Answer from the drawing. Dimensions are ordinates in mm from the lowest x, y and z of the part. Coordinates: 2 decimals unless noted, no trailing zeros. Write each loop counter-clockwise with the first axis right and the second up, starting at its lowest first coordinate (ties: lowest second). Pieces come first, ordered by that corner, then holes.
1) Each of these flat-tipped pins is pushed along its axis until it touches: pin 1 Ø1.5 at (y, z) = (1, 51.5) entering from +X; pin 2 Ø0.9 at (y, z) = (1.5, 51.5) entering from -X. Where does it stop, or does it pass through?
2) Find the intervals of material crossed by line 1 (X direction, y = 0.35, z = 23); line 2 (Z direction, x = 22.5, y = 0.25); line 3 (Z direction, x = 6.5, y = 1.55), in increasing order.
3) The part is cut by section A-A (x = 5.5). Determine the outline of the cut face in (y, z), then the cut area to 3 significant figures.
4) The part is cut by section B-B (z = 38). Determine the outline of the cut face in (x, y).
5) The part is cut by section C-C (y = 2.4). Determine the outline of the cut face in (x, z).
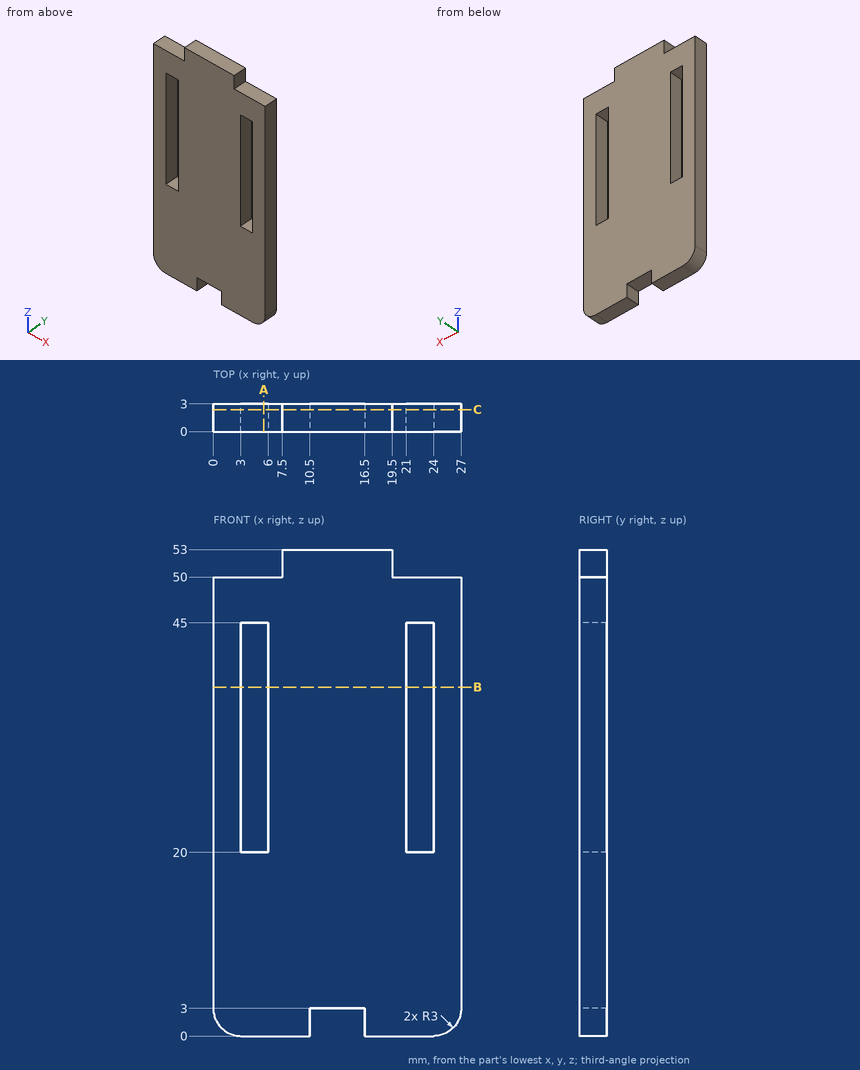
Reported:
1. pin 1: stops at x = 19.5
1. pin 2: stops at x = 7.5
2. line 1: x = 0 to 3, 6 to 21, 24 to 27
2. line 2: z = 0 to 20, 45 to 50
2. line 3: z = 0 to 50
3. outline: (0, 0) - (3, 0) - (3, 20) - (0, 20) - close; (0, 45) - (3, 45) - (3, 50) - (0, 50) - close
3. area: 75.0 mm2
4. outline: (0, 0) - (3, 0) - (3, 3) - (0, 3) - close; (6, 0) - (21, 0) - (21, 3) - (6, 3) - close; (24, 0) - (27, 0) - (27, 3) - (24, 3) - close
5. outline: (0, 3) arc R3 ccw to (3, 0) - (10.5, 0) - (10.5, 3) - (16.5, 3) - (16.5, 0) - (24, 0) arc R3 ccw to (27, 3) - (27, 50) - (19.5, 50) - (19.5, 53) - (7.5, 53) - (7.5, 50) - (0, 50) - close; hole (3, 20) - (6, 20) - (6, 45) - (3, 45) - close; hole (21, 20) - (24, 20) - (24, 45) - (21, 45) - close
